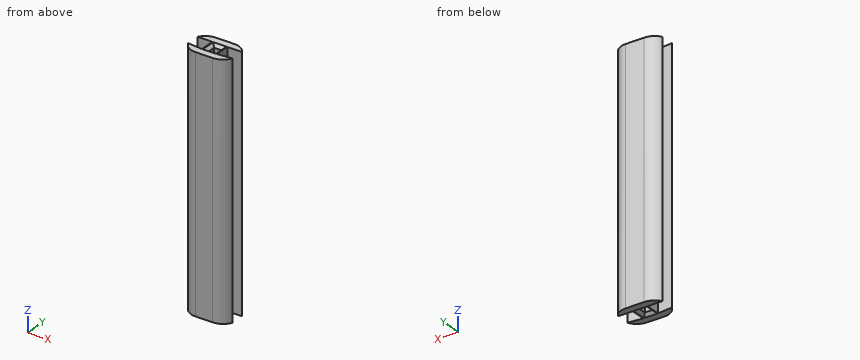
```python
from build123d import *

# Parameters (mm, degrees)
F1_DEPTH    = 83
F2_T1_DEPTH = 104.6506350946
F2_T3_DEPTH = 105.9128784748
F4_W        = 2.5
F4_H        = 3
F5_DEPTH    = 83.001
F6_SIZE     = 1


# Not quite as in the source:
# - a fillet or chamfer that OpenCascade refuses, or shapes differently, is made with other operations: its cross-section is extruded or revolved along the edge and cut away or added


with BuildPart() as f1:
    # F0 (on Top) → F1 (new body)
    with BuildSketch(Plane.XY):
        Polygon((0, -5), (0, 5), (-7.5, 5), (-7.5, 2.5), (-2.5, 2.5), (-2.5, -2.5), (-7.5, -2.5), (-7.5, -5), align=None)
        Polygon((-7.5, -2), (-7.5, -2.5), (-2.5, -2.5), align=None)
    extrude(amount=F1_DEPTH)

    # F2: fillet of radius 5 on 2 edges, made by hand

    # F2_s2 → F2_t1 (cut)
    with BuildSketch(Plane.XY.offset(-10.8253175473)):
        with BuildLine():
            ThreePointArc((-3.1698729811, 5), (-5.6698729811, 4.3301270189), (-7.5, 2.5))
            Line((-7.5, 2.5), (-7.5, 5))
            Line((-7.5, 5), (-3.1698729811, 5))
        make_face()
    extrude(amount=F2_T1_DEPTH, mode=Mode.SUBTRACT)

    # F2_s4 → F2_t3 (cut)
    with BuildSketch(Plane.XY.offset(-11.4564392374)):
        with BuildLine():
            ThreePointArc((-7.5, -2), (-5.6560370926, -4.1833001327), (-2.917424305, -5))
            Line((-2.917424305, -5), (-7.5, -5))
            Line((-7.5, -5), (-7.5, -2))
        make_face()
    extrude(amount=F2_T3_DEPTH, mode=Mode.SUBTRACT)

    # F3: F1 across face


with BuildPart() as f1_1:
    add(f1.part)
    add(f1.part.mirror(Plane(origin=(0, 0, 41.5), x_dir=(0, 1, 0), z_dir=(1, 0, 0))))

    # F4 (on face) → F5 (cut, through all)
    with BuildSketch(Plane.XY.offset(83)):
        Rectangle(F4_W, F4_H)
    extrude(amount=-F5_DEPTH, mode=Mode.SUBTRACT)

    # F6
    f6_edges = [f1_1.edges().sort_by_distance(p)[0] for p in [
        (1.25, 0, 83),
        (0, 1.5, 83),
        (-1.25, 0, 83),
        (0, -1.5, 83),
        (1.25, 0, 0),
        (0, -1.5, 0),
        (-1.25, 0, 0),
        (0, 1.5, 0),
    ]]
    chamfer(f6_edges, length=F6_SIZE)


solid = f1_1.part
```
Check sheet for the modelled part. Datum: model origin and axes. Units: mm. Round coordinates to 2 decimals unless told otherwise and drop trailing zeros. Loops run counter-clockwise (first coordinate to the right, second up) from the corner with the lowest first, then second, coordinate; pieces in that order, holes last. Notation, with made-up numbers: (-29.5, -14.75) - (19.5, -14.75) arc R32 cw to (19.5, 22.25) - close; hole circle Ø7 at (57, 86). An arc over 180 degrees is marked (long way). Answer as a JSON object with one key per item and string values. Group by question number.
Q1. Sectioned sample at C-C, the plane y = -0.25. Enter the section's corners in (x, z), plus the area to 4 significant figures.
Q2. Sectioned sample at B-B, the plane x = 0. Enter the section's corners in (y, z), plus the area to 3 significant figures.
Q3. Sectioned sample at D-D, the plane x = -6.5. Enter the section's corners in (y, z).
Q4. Gauge pin test, flat ends, axial feed: P1, Ø4, axis at y = 1, z = 52.5, coming from the -X side; P2, Ø0.9, axis at y = -0.5, z = 27, coming from the +X side; P3, Ø1.5, axis at x = 4, z = 11, coming from the -Y side. Record the tip position at first contact, or that the pin passes through.
Q5. Sectioned sample at A-A, the plane z = 50. Enter the section's corners in (x, y).
Q6. Scan lines: line 1 along X through (y, z) = (1, 55); line 2 along Y through (x, z) = (0.5, 76); line 3 along Y through (x, z) = (-6.5, 34.5). Record each from-to range of solid material in increasing order. Write a range as [from, to].
Solution:
{
 "1": {"outline": "(-2.5, 0) - (-2.25, 0) - (-1.25, 1) - (-1.25, 82) - (-2.25, 83) - (-2.5, 83) - close; (1.25, 1) - (2.25, 0) - (2.5, 0) - (2.5, 83) - (2.25, 83) - (1.25, 82) - close", "area": "205.5 mm²"},
 "2": {"outline": "(-5, 0) - (-2.5, 0) - (-1.5, 1) - (-1.5, 82) - (-2.5, 83) - (-5, 83) - close; (1.5, 1) - (2.5, 0) - (5, 0) - (5, 83) - (2.5, 83) - (1.5, 82) - close", "area": "579 mm²"},
 "3": {"outline": "(-3.49, 0) - (-2.1, 0) - (-2.1, 83) - (-3.49, 83) - close; (2.5, 0) - (3.73, 0) - (3.73, 83) - (2.5, 83) - close"},
 "4": {"P1": "stops at x = -7.5", "P2": "stops at x = 2.5", "P3": "stops at y = -4.99"},
 "5": {"outline": "(-7.5, -2) arc R5 ccw to (-2.92, -5) - (2.92, -5) arc R5 ccw to (7.5, -2) - (2.5, -2.5) - (2.5, 2.5) - (7.5, 2.5) arc R5 ccw to (3.17, 5) - (-3.17, 5) arc R5 ccw to (-7.5, 2.5) - (-2.5, 2.5) - (-2.5, -2.5) - close; hole (-1.25, -1.5) - (1.25, -1.5) - (1.25, 1.5) - (-1.25, 1.5) - close"},
 "6": {"line 1": "x = [-2.5, -1.25], [1.25, 2.5]", "line 2": "y = [-5, -1.5], [1.5, 5]", "line 3": "y = [-3.49, -2.1], [2.5, 3.73]"}
}
